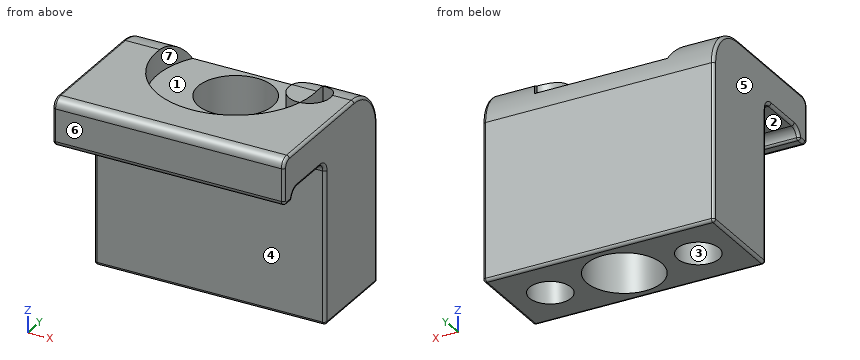
Autodesk Fusion 360 part; units mm, degrees
sketch "PhoneSupportTop" plane through (0, 0, 0) normal (1, 0, 0) x (0, 1, 0)
  line L0 (0, 0) -> (20, 0)
  line L1 (0, 33) -> (0, 0)
  line L2 (-2, 35) -> (-11, 35)
  line L3 (-13.4495, 33) -> (-15, 33)
  line L4 (-16, 34) -> (-16, 41)
  arc A0 (-11, 35) -> (-12.9596, 33.4) centre (-11, 33) ccw
  arc A1 (0, 33) -> (-2, 35) centre (-2, 33) ccw
  line L5 (-14, 43) -> (11, 43)
  line L6 (20, 0) -> (20, 34)
  arc A2 (20, 34) -> (11, 43) centre (11, 34) ccw
  arc A3 (-14, 43) -> (-16, 41) centre (-14, 41) ccw
  arc A4 (-13.4495, 33) -> (-12.9596, 33.4) centre (-13.4495, 33.5) ccw
  arc A5 (-16, 34) -> (-15, 33) centre (-15, 34) ccw
  point P0 (-13, 33)
  point P1 (-16, 33)
  point P2 (-16, 43)
  dimension "d3" = 20
  dimension "d7" = 4
  dimension "d8" = 3
  dimension "d10" = 2
  dimension "d11" = 9
  dimension "d13" = 34
  dimension "d14" = 27
  dimension "d15" = 10
  dimension "d16" = 9
  dimension "d17" = 2
  dimension "d18" = 0.5
  dimension "d19" = 1
extrude "Extrude1" add sketch "PhoneSupportTop" along normal mid plane 50
sketch "Sketch2" plane through (0, 0, 0) normal (0, 0, 1) x (1, 0, 0)
  line L0 (25, 20) -> (-25, 20) construction
  line L1 (-25, 20) -> (-25, 0) construction
  line L2 (-25, 0) -> (25, 0) construction
  line L3 (25, 0) -> (25, 20) construction
  line L4 (25, 10) -> (-25, 10) construction
  circle A0 centre (0, 10) radius 8.1
  circle A1 centre (16, 10) radius 4.5
  circle A2 centre (-16, 10) radius 4.5
  circle A3 centre (0, 10) radius 17
  dimension "d23" = 16.2
  dimension "d24" = 9
  dimension "d25" = 9
  dimension "d27" = 9
  dimension "d28" = 9
  dimension "d40" = 34
extrude "Extrude2" cut sketch "Sketch2" along normal blind 10 contours A1 A3 | A1 A3 | A2 A3 | A2 A3
extrude "Extrude3" cut sketch "Sketch2" along normal through all contours A0
extrude "Extrude4" cut sketch "Sketch2" against normal blind 5 from surface at 43 contours A0
fillet "Fillet1" radius 0.6 28 edges at (25, 20, 17) (25, 17.364, 40.364) (25, -1.5, 43) (25, -15.4142, 42.4142) (25, -16, 37.5) (25, -15.7071, 33.2929) (25, -14.2247, 33) (25, -13.1333, 33.1127) (25, -12.2649, 34.5492) (25, -6.5, 35) (25, -0.5858, 34.4142) (25, 0, 16.5) (25, 10, 0) (0, 0, 0) (-25, 0, 16.5) (-25, -0.5858, 34.4142) (-25, -6.5, 35) (-25, -12.2649, 34.5492) (-25, -13.1333, 33.1127) (-25, -14.2247, 33) (-25, -15.7071, 33.2929) (-25, -16, 37.5) (-25, -15.4142, 42.4142) (-25, -1.5, 43) (-25, 17.364, 40.364) (-25, 20, 17) (-25, 10, 0) (0, 20, 0)
extrude "Extrude5" cut sketch "Sketch2" against normal blind 5 from surface at 43 contours A1 A3 | A1 A2 A3 | A2 A3 picked at (18.0788, 10.9415) picked at (-15.34, 11.5418)
equation "PhoneSupportThickness = 50 mm"
equation "d21 = PhoneSupportThickness / 2"
equation "d23 = 16 mm + 2 * Tolerance"
equation "Tolerance = 0.1 mm"
The model under review builds one solid part; all positions refer to its coordinate system, in mm. Face numbers are marked on the shaded views. A direction names the side the tool comes from. Give positions to 0.01 mm unless a question says otherwise; leave off trailing zeros. Order: outer loops, then holes, each group sorted by start corner. A loop starts at its lowest first (then second) coordinate and runs counter-clockwise, first axis right, second up. Notation, with made-up numbers: M 8.25,49.5 L 56.25,49.5 A23 cw 56.25,66.5 Z; hole C 80.5,-22 d8. An arc over 180 degrees is marked long. One line per question, with ' | ' between items. Start each with the question number.
1) Consider section A-A, the plane x = 0. Give the boundary of the cut face in (y, z).
2) For the marked faces 1, 2, 3 and 4, list the 3-axis set-ups (+Z, -Z, +X, -X, +Y, -Y) from which the entire face can be reached by the end or side of a thin tool; tool diameter is ignored.
3) Wall thickness on L1, parallel to X at y = 10, z = 39.1; L2, parallel to Y at x = 0, z = 28; L3, parallel to Y at x = -16, z = 5: over which ranges is each line inside the solid? List them lowest first. Write a range as from..to.
4) Clearance check with flat-ended pins moving along their axes: P1, Ø3, axis at x = 18.5, z = 14, coming from the -Y side; P2, Ø13, axis at x = -7, y = 11.5, coming from the +Z side; P3, Ø4.5, axis at x = -5, y = -7.5, coming from the -Z side; P4, Ø13, axis at x = 0, y = 10, coming from the -Z side. State where each tip first meets the part, or that it passes through.
5) Consider section D-D, the plane z = 17.5. Give the boundary of the cut face in (x, y).
6) Consider section C-C, the plane y = 10. Give the boundary of the cut face in (x, z), then the cut area to 3 significant figures.
7) Mouldability with a two-part tool opening along Y and no side actions: class the marked faces 5, 6 and 7 as pulls with the +Y half, pulls with the -Y half, needs draft (parallel to the pull), parting line crosses it, or undercut.
8) Consider section B-B, the plane z = 8.5. Give the boundary of the cut face in (x, y).
Found:
1) outline: M -16,34 A1 ccw -15,33 L -13.45,33 A0.5 ccw -12.96,33.4 A2 cw -11,35 L -2,35 A2 cw 0,33 L 0,0.6 A0.6 ccw 0.6,0 L 1.9,0 L 1.9,38 L -7,38 L -7,43 L -14,43 A2 ccw -16,41 Z; M 18.1,0 L 19.4,0 A0.6 ccw 20,0.6 L 20,34 A9 ccw 19.06,38 L 18.1,38 Z
2) face 1: +Z | face 2: -Z, +X, -X | face 3: -Z | face 4: -Z, +X, -X, -Y
3) L1: x = -25..-17, 11.5..17, 20.5..25 | L2: y = 0..1.9, 18.1..20 | L3: y = 0..5.5, 14.5..20
4) P1: stops at y = 0 | P2: stops at z = 38 | P3: stops at z = 35 | P4: passes through
5) outline: M -25,0.6 A0.6 ccw -24.4,0 L 24.4,0 A0.6 ccw 25,0.6 L 25,19.4 A0.6 ccw 24.4,20 L -24.4,20 A0.6 ccw -25,19.4 Z; hole C 0,10 d16.2
6) outline: M -25,0.6 A0.6 ccw -24.4,0 L -20.5,0 L -20.5,10 L -11.5,10 L -11.5,0 L -8.1,0 L -8.1,38 L -17,38 L -17,43 L -24.4,43 A0.6 ccw -25,42.4 Z; M 8.1,0 L 11.5,0 L 11.5,10 L 20.5,10 L 20.5,0 L 24.4,0 A0.6 ccw 25,0.6 L 25,42.4 A0.6 ccw 24.4,43 L 20.5,43 L 20.5,38 L 17,38 L 17,43 L 11.5,43 L 11.5,38 L 8.1,38 Z | area: 1,190 mm²
7) face 5: needs draft | face 6: pulls with the -Y half | face 7: undercut
8) outline: M -25,0.6 A0.6 ccw -24.4,0 L 24.4,0 A0.6 ccw 25,0.6 L 25,19.4 A0.6 ccw 24.4,20 L -24.4,20 A0.6 ccw -25,19.4 Z; hole C -16,10 d9; hole C 0,10 d16.2; hole C 16,10 d9
